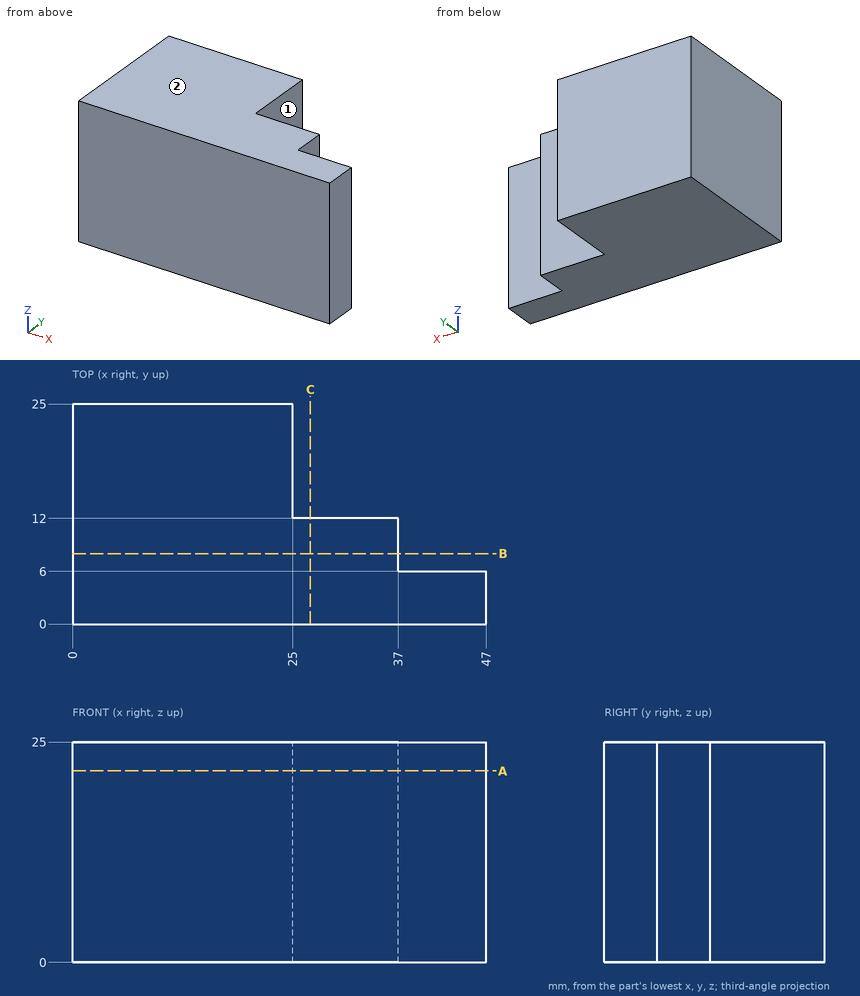
Answer from the drawing. Dimensions are ordinates in mm from the lowest x, y and z of the part. A direction names the side the tool comes from. Coordinates: 2 decimals unless noted, no trailing zeros. Order: outer loops, then holes, each group sorted by start corner. A loop starts at its lowest first (then second) coordinate and runs counter-clockwise, first axis right, second up. Notation, with made-up numbers: (75.25, -35) - (100.25, -35) arc R16 ccw to (100.25, -12) - close; hole circle Ø1 at (-23.75, 4.5). An arc over 180 degrees is marked (long way). Put each result on its own line as item: value. Start each with the question number.
1) Find section B-B (y = 8). Give the vertices of the cut face in (x, z), plus the area to 3 significant figures.
2) Flat-ended cylindrical pins translate along their axes: pin 1 (5 mm diameter, centred on x = 42.5, z = 11.5, fed in from +Y); pin 2 (6 mm diameter, centred on x = 41.5, y = 14, fed in from +Z); pin 3 (4 mm diameter, centred on y = 17.5, z = 17, fed in from +X); pin 4 (3 mm diameter, centred on y = 11, z = 19, fed in from +X). Find the tip coordinate at first contact, or state that the pin passes through.
3) Find the intervals of material crossed by line 1 (X direction, y = 11.5, z = 3); line 2 (X direction, y = 13, z = 23.75); line 3 (Y direction, x = 30.5, z = 9), in increasing order. Write a range as from..to.
4) Find section A-A (z = 21.75). Give the vertices of the cut face in (x, y), plus the area to 3 significant figures.
5) For the marked faces 1 and 2, determine the directions among +Z, -Z, +X, -X, +Y, -Y from which every point of the face is accessible in a straight line to the end or side of a thin tool.
6) Find section C-C (x = 27). Give the vertices of the cut face in (y, z), plus the area to 3 significant figures.
Results list:
1. outline: (0, 0) - (37, 0) - (37, 25) - (0, 25) - close
1. area: 925 mm^2
2. pin 1: stops at y = 6
2. pin 2: passes through
2. pin 3: stops at x = 25
2. pin 4: stops at x = 37
3. line 1: x = 0..37
3. line 2: x = 0..25
3. line 3: y = 0..12
4. outline: (0, 0) - (47, 0) - (47, 6) - (37, 6) - (37, 12) - (25, 12) - (25, 25) - (0, 25) - close
4. area: 829 mm^2
5. face 1: +Z, -Z, +X, +Y
5. face 2: +Z, +X, -X, +Y, -Y
6. outline: (0, 0) - (12, 0) - (12, 25) - (0, 25) - close
6. area: 300 mm^2
